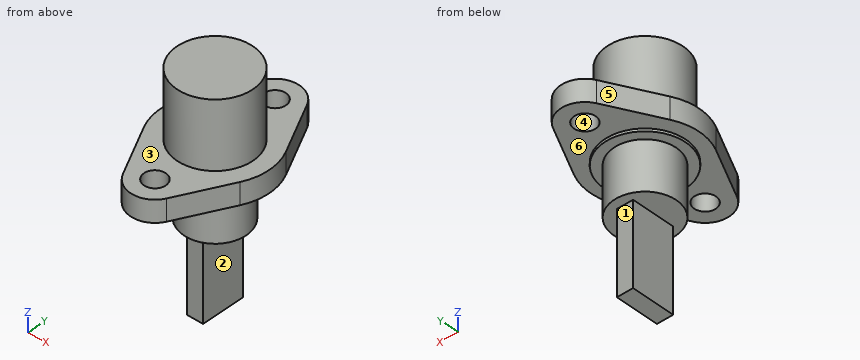
```python
from build123d import *

# Parameters (mm, degrees)
SKETCH1_R           = 2
BOSS_EXTRUDE1_DEPTH = 4
SKETCH2_R           = 7
BOSS_EXTRUDE2_DEPTH = 12.3
SKETCH3_R           = 7.5
BOSS_EXTRUDE3_DEPTH = 0.5
SKETCH4_W           = 3
SKETCH4_H           = 8
BOSS_EXTRUDE4_DEPTH = 24.2
SKETCH5_R           = 5.75
BOSS_EXTRUDE5_DEPTH = 9


with BuildPart() as part:
    # Sketch1 → Boss-Extrude1 (new body)
    with BuildSketch(Plane.XY):
        with BuildLine():
            ThreePointArc((-3.999511648, -14.062500079), (-8.7e-08, -16.5), (3.999511568, -14.062500234))
            Line((3.999511568, -14.062500234), (8.887803753, -4.583333333))
            ThreePointArc((8.887803753, -4.583333333), (10, 0), (8.887803753, 4.583333333))
            Line((8.887803753, 4.583333333), (3.999511579, 14.062500214))
            ThreePointArc((3.999511579, 14.062500214), (-6.7e-08, 16.5), (-3.99951164, 14.062500095))
            Line((-3.99951164, 14.062500095), (-8.887803753, 4.583333333))
            ThreePointArc((-8.887803753, 4.583333333), (-10, 0), (-8.887803753, -4.583333333))
            Line((-8.887803753, -4.583333333), (-3.999511648, -14.062500079))
        make_face()
        with Locations((0, -12)):
            Circle(SKETCH1_R, mode=Mode.SUBTRACT)
        with Locations((0, 12)):
            Circle(SKETCH1_R, mode=Mode.SUBTRACT)
    extrude(amount=BOSS_EXTRUDE1_DEPTH)

    # Sketch2 → Boss-Extrude2 (add)
    with BuildSketch(Plane.XY.offset(4)):
        Circle(SKETCH2_R)
    extrude(amount=BOSS_EXTRUDE2_DEPTH)

    # Sketch3 → Boss-Extrude3 (add)
    with BuildSketch(Plane(origin=(0, 0, 0), x_dir=(-1, 0, 0), z_dir=(0, 0, -1))):
        with Locations(Location((0, 0, 0), (0, 0, 180))):
            Circle(SKETCH3_R)
    extrude(amount=BOSS_EXTRUDE3_DEPTH)

    # Sketch4 → Boss-Extrude4 (add)
    with BuildSketch(Plane(origin=(0, 0, -0.5), x_dir=(-1, 0, 0), z_dir=(0, 0, -1))):
        Rectangle(SKETCH4_W, SKETCH4_H)
    extrude(amount=BOSS_EXTRUDE4_DEPTH)

    # Sketch5 → Boss-Extrude5 (add)
    with BuildSketch(Plane(origin=(0, 0, -0.5), x_dir=(-1, 0, 0), z_dir=(0, 0, -1))):
        Circle(SKETCH5_R)
    extrude(amount=BOSS_EXTRUDE5_DEPTH)


solid = part.part
```
Input: part model. Units: mm. Frame: model coordinates. Face numbers are marked on the shaded views. A direction names the side the tool comes from. Give positions to 0.01 mm unless a question says otherwise; leave off trailing zeros. Order: outer loops, then holes, each group sorted by start corner. A loop starts at its lowest first (then second) coordinate and runs counter-clockwise, first axis right, second up.
1. Section C-C on y = 0. Return the cut outline in (x, z), and give its area (3 significant figures).
Derived:
outline: (-10, 0) - (-7.5, 0) - (-7.5, -0.5) - (-5.75, -0.5) - (-5.75, -9.5) - (-1.5, -9.5) - (-1.5, -24.7) - (1.5, -24.7) - (1.5, -9.5) - (5.75, -9.5) - (5.75, -0.5) - (7.5, -0.5) - (7.5, 0) - (10, 0) - (10, 4) - (7, 4) - (7, 16.3) - (-7, 16.3) - (-7, 4) - (-10, 4) - close
area: 409 mm2
2. Section D-D on z = -21. Return the cut outline in (x, y).
Derived:
outline: (-1.5, -4) - (1.5, -4) - (1.5, 4) - (-1.5, 4) - close
3. Section A-A on x = 0. Return the cut outline in (y, z).
Derived:
outline: (-16.5, 0) - (-14, 0) - (-14, 4) - (-16.5, 4) - close; (-10, 0) - (-7.5, 0) - (-7.5, -0.5) - (-5.75, -0.5) - (-5.75, -9.5) - (-4, -9.5) - (-4, -24.7) - (4, -24.7) - (4, -9.5) - (5.75, -9.5) - (5.75, -0.5) - (7.5, -0.5) - (7.5, 0) - (10, 0) - (10, 4) - (7, 4) - (7, 16.3) - (-7, 16.3) - (-7, 4) - (-10, 4) - close; (14, 0) - (16.5, 0) - (16.5, 4) - (14, 4) - close
4. Reachability of the marked faces 1, 2 and 3 from +Z, -Z, +X, -X, +Y, -Y: full face, straight path, thin tool, end or side. Return the list, or none.
Derived:
face 1: -Z, +X, -X, +Y
face 2: -Z, +X, +Y, -Y
face 3: +Z
5. Material intervals for L1, parallel to Y at x = 0, z = 3; L2, parallel to Z at x = -8.5, y = 2; L3, parallel to Z at x = -3.25, y = -5.5, sorted ascending.
Derived:
L1: y = -16.5 to -14, -10 to 10, 14 to 16.5
L2: z = 0 to 4
L3: z = -0.5 to 16.3
6. Section B-B on y = 11. Return the cut outline in (x, z).
Derived:
outline: (-5.58, 0) - (-1.73, 0) - (-1.73, 4) - (-5.58, 4) - close; (1.73, 0) - (5.58, 0) - (5.58, 4) - (1.73, 4) - close
7. Pin query (flat end, axial travel): pin 1 (5 mm diameter, centred on x = 0.5, y = -9, fed in from -Z); pin 2 (4 mm diameter, centred on y = -0.5, z = -19, fed in from -X); pin 3 (12 mm diameter, centred on y = 0, z = 12, fed in from -X); pin 4 (2 mm diameter, centred on x = -3, z = -14, fed in from +Y). Return the tip coordinate at first contact, or that it passes through.
Derived:
pin 1: stops at z = -0.5
pin 2: stops at x = -1.5
pin 3: stops at x = -7
pin 4: passes through
8. Mould query, pull axis Y, two halves, no side actions, for the marked faces 4, 5 and 6. Classes: released by +Y, released by -Y, zero draft, split by the parting line, or undercut.
Derived:
face 4: undercut
face 5: released by +Y
face 6: zero draft
